Read the model definition and answer for the solid it produces. Units are mm, in the model's axes. Round coordinates to 2 decimals unless told otherwise and drop trailing zeros. Loops run counter-clockwise (first coordinate to the right, second up) from the corner with the lowest first, then second, coordinate; pieces in that order, holes last. Notation, with made-up numbers: (-24, -24) - (27, -24) arc R9 ccw to (27, -17) - close; hole circle Ø9 at (23.5, 24). An arc over 180 degrees is marked (long way). Use one line per item in the form item = value. Start each with the question number.
```python
from build123d import *

# Parameters (mm, degrees)
CROQUIS1_R              = 75
SALIENTE_EXTRUIR1_DEPTH = 3
CROQUIS4_W              = 35
CROQUIS4_H              = 23
CORTAR_EXTRUIR9_DEPTH   = 107.108435103
CROQUIS5_W              = 31
CROQUIS5_H              = 56
CROQUIS5_W_2            = 25
CORTAR_EXTRUIR10_DEPTH  = 107.108435103
CROQUIS6_W              = 29.5
CROQUIS6_H              = 35
CORTAR_EXTRUIR11_DEPTH  = 91.188691087
CROQUIS7_R              = 1.59
CORTAR_EXTRUIR12_DEPTH  = 91.188691087
CORTAR_EXTRUIR13_DEPTH  = 91.188691087
CROQUIS9_R              = 7
CROQUIS9_R_2            = 2
CORTAR_EXTRUIR15_DEPTH  = 90.38679992
CROQUIS10_W             = 100
CROQUIS10_H             = 10
CROQUIS10_R             = 2
SALIENTE_EXTRUIR2_DEPTH = 3
CROQUIS11_R             = 1.5
CORTAR_EXTRUIR16_DEPTH  = 90.38679992
CROQUIS12_W             = 100
CROQUIS12_H             = 103
CORTAR_EXTRUIR17_DEPTH  = 90.38679992


with BuildPart() as part:
    # Croquis1 → Saliente-Extruir1 (new body)
    with BuildSketch(Plane(origin=(0, 0, 0), x_dir=(1, 0, 0), z_dir=(0, 1, 0))):
        with Locations(Location((0, 0, 0), (0, 0, 270))):
            Circle(CROQUIS1_R)
    extrude(amount=SALIENTE_EXTRUIR1_DEPTH)

    # Croquis4 → Cortar-Extruir9 (cut, through all)
    with BuildSketch(Plane(origin=(0, 3, 0), x_dir=(1, 0, 0), z_dir=(0, 1, 0))):
        with Locations((0, -18.5)):
            Rectangle(CROQUIS4_W, CROQUIS4_H)
    extrude(amount=-CORTAR_EXTRUIR9_DEPTH, mode=Mode.SUBTRACT)

    # Croquis5 → Cortar-Extruir10 (cut, through all)
    with BuildSketch(Plane(origin=(0, 3, 0), x_dir=(1, 0, 0), z_dir=(0, 1, 0))):
        Polygon((-50, 55), (0, 55), (0, 77), (-53, 77), (-53, 55), align=None)
        Polygon((0, 77), (0, 55), (50, 55), (53, 55), (53, 77), align=None)
        Polygon((-50, 0), (-50, 55), (-53, 55), (-81, 55), (-81, 0), align=None)
        Polygon((53, 55), (50, 55), (50, 0), (75, 0), (75, 55), align=None)
        with Locations((-65.5, -28)):
            Rectangle(CROQUIS5_W, CROQUIS5_H)
        with Locations((62.5, -28)):
            Rectangle(CROQUIS5_W_2, CROQUIS5_H)
    extrude(amount=-CORTAR_EXTRUIR10_DEPTH, mode=Mode.SUBTRACT)

    # Croquis6 → Cortar-Extruir11 (cut, through all)
    with BuildSketch(Plane(origin=(0, 3, 0), x_dir=(1, 0, 0), z_dir=(0, 1, 0))):
        with Locations((-35.25, -20.5)):
            Rectangle(CROQUIS6_W, CROQUIS6_H)
        with Locations((35.25, -20.5)):
            Rectangle(CROQUIS6_W, CROQUIS6_H)
    extrude(amount=-CORTAR_EXTRUIR11_DEPTH, mode=Mode.SUBTRACT)

    # Croquis7 → Cortar-Extruir12 (cut, through all)
    with BuildSketch(Plane(origin=(0, 3, 0), x_dir=(1, 0, 0), z_dir=(0, 1, 0))):
        with Locations(Location((-46.52, 47.87, 0), (0, 0, 270))):
            Circle(CROQUIS7_R)
        with Locations(Location((-40.17, -0.46, 0), (0, 0, 270))):
            Circle(CROQUIS7_R)
        with Locations(Location((36.03, 47.8, 0), (0, 0, 270))):
            Circle(CROQUIS7_R)
        with Locations(Location((34.76, -0.46, 0), (0, 0, 270))):
            Circle(CROQUIS7_R)
    extrude(amount=-CORTAR_EXTRUIR12_DEPTH, mode=Mode.SUBTRACT)

    # Croquis8 → Cortar-Extruir13 (cut, through all)
    with BuildSketch(Plane(origin=(0, 3, 0), x_dir=(1, 0, 0), z_dir=(0, 1, 0))):
        with BuildLine():
            ThreePointArc((-12, -74.033776076), (-6.019418341, -74.758053766), (0, -75))
            Line((0, -75), (0, -45))
            Line((0, -45), (-12, -45))
            Line((-12, -45), (-12, -74.033776076))
        make_face()
        with BuildLine():
            Line((0, -45), (0, -75))
            ThreePointArc((0, -75), (6.019418341, -74.758053766), (12, -74.033776076))
            Line((12, -74.033776076), (12, -45))
            Line((12, -45), (0, -45))
        make_face()
    extrude(amount=-CORTAR_EXTRUIR13_DEPTH, mode=Mode.SUBTRACT)

    # Croquis9 → Cortar-Extruir15 (cut, through all)
    with BuildSketch(Plane(origin=(0, 3, 0), x_dir=(1, 0, 0), z_dir=(0, 1, 0))):
        with Locations(Location((-30, -55.493776076, 0), (0, 0, 270))):
            Circle(CROQUIS9_R)
        with Locations(Location((30, -55.493776076, 0), (0, 0, 90))):
            Circle(CROQUIS9_R)
        with Locations(Location((-47.5, -54.5, 0), (0, 0, 270))):
            Circle(CROQUIS9_R_2)
        with Locations(Location((46.5, -54.5, 0), (0, 0, 270))):
            Circle(CROQUIS9_R_2)
    extrude(amount=-CORTAR_EXTRUIR15_DEPTH, mode=Mode.SUBTRACT)

    # Croquis10 → Saliente-Extruir2 (add)
    with BuildSketch(Plane(origin=(0, 3, 0), x_dir=(1, 0, 0), z_dir=(0, 1, 0))):
        with Locations((0, 60)):
            Rectangle(CROQUIS10_W, CROQUIS10_H)
        with Locations(Location((-45, 60, 0), (0, 0, 270))):
            Circle(CROQUIS10_R, mode=Mode.SUBTRACT)
        with Locations(Location((45, 60, 0), (0, 0, 270))):
            Circle(CROQUIS10_R, mode=Mode.SUBTRACT)
    extrude(amount=-SALIENTE_EXTRUIR2_DEPTH)

    # Croquis11 → Cortar-Extruir16 (cut, through all)
    with BuildSketch(Plane(origin=(0, 3, 0), x_dir=(1, 0, 0), z_dir=(0, 1, 0))):
        with Locations(Location((-16.5, -49, 0), (0, 0, 270))):
            Circle(CROQUIS11_R)
        with Locations(Location((-16.5, -63, 0), (0, 0, 270))):
            Circle(CROQUIS11_R)
        with Locations(Location((16.5, -63, 0), (0, 0, 90))):
            Circle(CROQUIS11_R)
        with Locations(Location((16.5, -49, 0), (0, 0, 90))):
            Circle(CROQUIS11_R)
    extrude(amount=-CORTAR_EXTRUIR16_DEPTH, mode=Mode.SUBTRACT)

    # Croquis12 → Cortar-Extruir17 (cut, through all)
    with BuildSketch(Plane(origin=(0, 3, 0), x_dir=(1, 0, 0), z_dir=(0, 1, 0))):
        with Locations((0, 13.5)):
            Rectangle(CROQUIS12_W, CROQUIS12_H)
    extrude(amount=-CORTAR_EXTRUIR17_DEPTH, mode=Mode.SUBTRACT)


solid = part.part
```
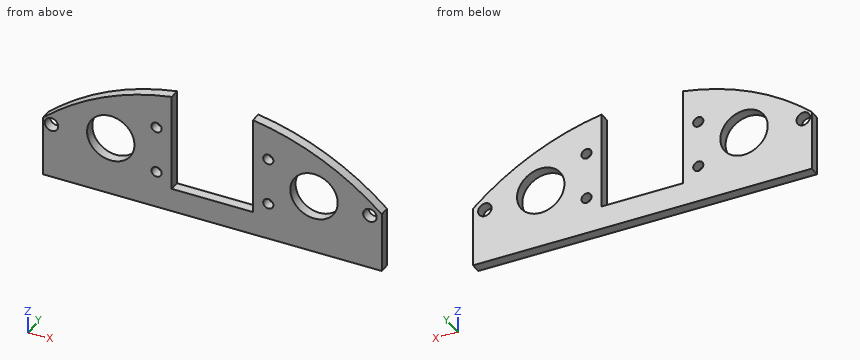
1) Straight lines are drawn through the part: line 1 (X direction, y = 0.85, z = 63); line 2 (X direction, y = 1.15, z = 54.5); line 3 (X direction, y = 0.8, z = 60.5). For each, find the intervals that lie inside material, in ascending order. Write a range as from..to.
2) A cutting plane is placed at A-A on z = 46. Write down the section's boundary in (x, y), plus the area to 3 significant figures.
3) Flat-ended cylindrical pins translate along their axes: pin 1 (1.8 mm diameter, centred on x = -16.5, z = 49, fed in from +Y); pin 2 (1 mm diameter, centred on y = 2.5, z = 64.5, fed in from -X); pin 3 (1 mm diameter, centred on x = 28, y = 0.5, fed in from +Z). Find the tip coordinate at first contact, or state that the pin passes through.
4) A cutting plane is placed at C-C on x = 16.5. Write down the section's boundary in (y, z), plus the area to 3 significant figures.
5) A cutting plane is placed at B-B on y = 2.5. Count the separate pieces of the cut face and the enclosed holes in it, plus the area to 3 significant figures.
6) A cutting plane is placed at D-D on z = 54.5. Write down the section's boundary in (x, y).
Checks:
q1.line_1 = -40.69..-18, -15..-12, 12..15, 18..40.69
q1.line_2 = -50..-49.5, -45.5..-36.93, -23.07..-12, 12..23.07, 36.93..44.5, 48.5..50
q1.line_3 = -44.33..-34.89, -25.11..-12, 12..25.11, 34.89..44.33
q2.outline = (-50, 0) - (-12, 0) - (-12, 3) - (-50, 3) - close; (12, 0) - (50, 0) - (50, 3) - (12, 3) - close
q2.area = 228 mm²
q3.pin_1 = through
q3.pin_2 = -39.1
q3.pin_3 = 69.78
q4.outline = (0, 38) - (3, 38) - (3, 47.5) - (0, 47.5) - close; (0, 50.5) - (3, 50.5) - (3, 61.5) - (0, 61.5) - close; (0, 64.5) - (3, 64.5) - (3, 73.16) - (0, 73.16) - close
q4.area = 87.5 mm²
q5.separate_pieces = 1
q5.enclosed_holes = 8
q5.area = 2,030 mm²
q6.outline = (-50, 0) - (-49.5, 0) - (-49.5, 3) - (-50, 3) - close; (-45.5, 0) - (-36.93, 0) - (-36.93, 3) - (-45.5, 3) - close; (-23.07, 0) - (-12, 0) - (-12, 3) - (-23.07, 3) - close; (12, 0) - (23.07, 0) - (23.07, 3) - (12, 3) - close; (36.93, 0) - (44.5, 0) - (44.5, 3) - (36.93, 3) - close; (48.5, 0) - (50, 0) - (50, 3) - (48.5, 3) - close
